```python
from build123d import *

# Parameters (mm, degrees)
SKETCH050_R      = 2
SKETCH050_R_2    = 1.5
EXTRUDE038_DEPTH = 6.5
EXTRUDE039_DEPTH = 45
SKETCH052_R      = 2
SKETCH052_R_2    = 1.5
EXTRUDE040_DEPTH = 6.5


with BuildPart() as extrude038:
    # Sketch050 → Extrude038 (new body)
    with BuildSketch(Plane.XY):
        with BuildLine():
            Line((-15, 22.5), (-6.25, 22.5))
            Line((-6.25, 25.100357), (-6.25, 22.5))
            ThreePointArc((6.25, 25.100357), (0, 31.350357), (-6.25, 25.100357))
            Line((6.25, 25.100357), (6.25, 22.5))
            Line((6.25, 22.5), (15, 22.5))
            Line((15, 22.5), (15, -22.5))
            Line((15, -22.5), (3.522198, -22.5))
            ThreePointArc((-3.522198, -22.5), (0, -24.962903), (3.522198, -22.5))
            Line((-3.522198, -22.5), (-15, -22.5))
            Line((-15, -22.5), (-15, 22.5))
        make_face()
        with Locations((0, 25.100357)):
            Circle(SKETCH050_R, mode=Mode.SUBTRACT)
        with Locations((0, -20.5)):
            Circle(SKETCH050_R_2, mode=Mode.SUBTRACT)
    extrude(amount=-EXTRUDE038_DEPTH)


with BuildPart() as extrude038_1:
    # Extrude038 placement: moved
    add(extrude038.part.moved(Location((0, 0, -34.999))))


with BuildPart() as extrude039:
    # Sketch051 (on Face13 of Extrude038) → Extrude039 (new body)
    with BuildSketch(Plane(origin=(0, 0, -41.499), x_dir=(1, 0, 0), z_dir=(0, 0, -1))):
        with BuildLine():
            ThreePointArc((-7.5, 15), (-12.803301, 12.803301), (-15, 7.5))
            Line((-15, -7.5), (-15, 7.5))
            ThreePointArc((-15, -7.5), (-12.803301, -12.803301), (-7.5, -15))
            Line((7.5, -15), (-7.5, -15))
            ThreePointArc((7.5, -15), (12.803301, -12.803301), (15, -7.5))
            Line((15, 7.5), (15, -7.5))
            ThreePointArc((15, 7.5), (12.803301, 12.803301), (7.5, 15))
            Line((-7.5, 15), (7.5, 15))
        make_face()
    extrude(amount=EXTRUDE039_DEPTH)


with BuildPart() as actuator_base:
    # Sketch052 → Extrude040 (new body)
    with BuildSketch(Plane.XY):
        with BuildLine():
            Line((-15, 22.5), (-6.25, 22.5))
            Line((-6.25, 25.100357), (-6.25, 22.5))
            ThreePointArc((6.25, 25.100357), (0, 31.350357), (-6.25, 25.100357))
            Line((6.25, 25.100357), (6.25, 22.5))
            Line((6.25, 22.5), (15, 22.5))
            Line((15, 22.5), (15, -22.5))
            Line((15, -22.5), (3.522198, -22.5))
            ThreePointArc((-3.522198, -22.5), (0, -24.962903), (3.522198, -22.5))
            Line((-3.522198, -22.5), (-15, -22.5))
            Line((-15, -22.5), (-15, 22.5))
        make_face()
        with Locations((0, 25.100357)):
            Circle(SKETCH052_R, mode=Mode.SUBTRACT)
        with Locations((0, -20.5)):
            Circle(SKETCH052_R_2, mode=Mode.SUBTRACT)
    extrude(amount=-EXTRUDE040_DEPTH)


with BuildPart() as actuator_base_1:
    # Extrude040 placement: moved
    add(actuator_base.part.moved(Location((0, 0, -86.499))))

    # Fusion017: union Extrude038, Extrude039
    add(extrude038_1.part)
    add(extrude039.part)


solid = actuator_base_1.part
```
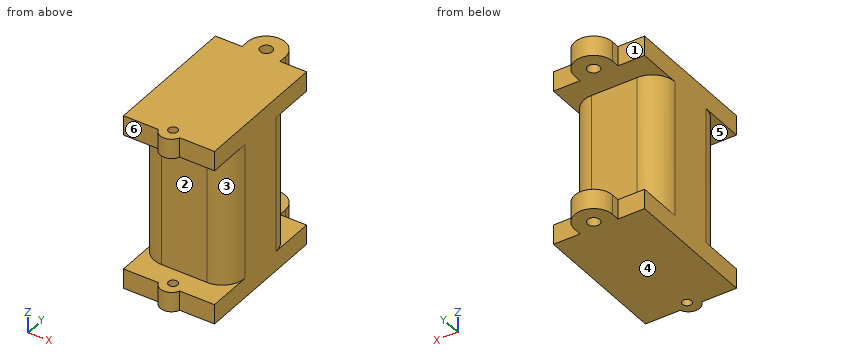
Check sheet for the modelled part. Datum: model origin and axes. Units: mm. Face numbers are marked on the shaded views. A direction names the side the tool comes from. Give positions to 0.01 mm unless a question says otherwise; leave off trailing zeros. Order: outer loops, then holes, each group sorted by start corner. A loop starts at its lowest first (then second) coordinate and runs counter-clockwise, first axis right, second up. Notation, with made-up numbers: M 24.5,33 L 63.5,33 A18 cw 63.5,38 Z; hole C -38,11.25 d1. An arc over 180 degrees is marked long. Answer in a Markdown table with one row per item. Add a question column.
Q1. Sectioned sample at D-D, the plane x = 11. Record the boundary of the cut face in (y, z), and give its area (3 significant figures).
Q2. Sectioned sample at C-C, the plane z = -49.5. Record the boundary of the cut face in (x, y).
Q3. Release check for a two-part mould opening along Z. For the marked faces 4, 5 and 6 record: released by +Z, released by -Z, zero draft, split by the parting line, or undercut.
Q4. Gauge pin test, flat ends, axial feed: pin 1 Ø12 at (x, z) = (2.5, -62.5) entering from -Y; pin 2 Ø3 at (x, z) = (-11.5, -88.5) entering from +Y; pin 3 Ø1.3 at (y, z) = (24, -89) entering from -X. Record the tip position at first contact, or that the pin passes through.
Q5. Sectioned sample at B-B, the plane x = 0. Record the boundary of the cut face in (y, z), and give its area (3 significant figures).
Q6. Thickness scan on L1, parallel to Y at x = 0, z = -36.5; L2, parallel to Z at x = -7.5, y = -19.5; L3, parallel to Y at x = 0.5, z = -68.5. Record the ranges inside material, lowest first.
Q7. Access from +Z, -Z, +X, -X, +Y, -Y to the whole of each face (thin tool, end or side, straight path). Record for the marked faces 1, 2 and 3.
Q8. Sectioned sample at A-A, the plane y = -20.5. Record the boundary of the cut face in (x, z).
Verdict:
| question | item | result |
|---|---|---|
| 1 | outline | M -22.5,-93 L 22.5,-93 L 22.5,-86.5 L 14.13,-86.5 L 14.13,-41.5 L 22.5,-41.5 L 22.5,-35 L -22.5,-35 L -22.5,-41.5 L -14.13,-41.5 L -14.13,-86.5 L -22.5,-86.5 Z |
| 1 | area | 1,860 mm² |
| 2 | outline | M -15,-7.5 A7.5 ccw -7.5,-15 L 7.5,-15 A7.5 ccw 15,-7.5 L 15,7.5 A7.5 ccw 7.5,15 L -7.5,15 A7.5 ccw -15,7.5 Z |
| 3 | face 4 | released by -Z |
| 3 | face 5 | undercut |
| 3 | face 6 | zero draft |
| 4 | pin 1 | y = -15 |
| 4 | pin 2 | y = 22.5 |
| 4 | pin 3 | x = -6.25 |
| 5 | outline | M -24.96,-93 L -22,-93 L -22,-86.5 L -24.96,-86.5 Z; M -24.96,-41.5 L -22,-41.5 L -22,-35 L -24.96,-35 Z; M -19,-93 L 23.1,-93 L 23.1,-86.5 L 15,-86.5 L 15,-41.5 L 23.1,-41.5 L 23.1,-35 L -19,-35 L -19,-41.5 L -15,-41.5 L -15,-86.5 L -19,-86.5 Z; M 27.1,-93 L 31.35,-93 L 31.35,-86.5 L 27.1,-86.5 Z; M 27.1,-41.5 L 31.35,-41.5 L 31.35,-35 L 27.1,-35 Z |
| 5 | area | 1,990 mm² |
| 6 | L1 | -24.96 to -22, -19 to 23.1, 27.1 to 31.35 |
| 6 | L2 | -93 to -86.5, -41.5 to -35 |
| 6 | L3 | -15 to 15 |
| 7 | face 1 | +Z, -Z, -X, +Y |
| 7 | face 2 | +X, -X, -Y |
| 7 | face 3 | +X, -Y |
| 8 | outline | M -15,-93 L -1.5,-93 L -1.5,-86.5 L -15,-86.5 Z; M -15,-41.5 L -1.5,-41.5 L -1.5,-35 L -15,-35 Z; M 1.5,-93 L 15,-93 L 15,-86.5 L 1.5,-86.5 Z; M 1.5,-41.5 L 15,-41.5 L 15,-35 L 1.5,-35 Z |
